```python
from build123d import *

# Parameters (mm, degrees)
F0_W     = 73.152
F0_H     = 76.2
F1_DEPTH = 22.352
F2_SIZE  = 25.4
F3_SIZE  = 6.35


with BuildPart() as f1:
    # F0 (on Right) → F1 (new body)
    with BuildSketch(Plane.YZ):
        with Locations((36.576, -38.1)):
            Rectangle(F0_W, F0_H)
    extrude(amount=F1_DEPTH)

    # F2
    f2_edges = [f1.edges().sort_by_distance(p)[0] for p in [
        (11.176, 0, -76.2),
        (11.176, 73.152, -76.2),
    ]]
    chamfer(f2_edges, length=F2_SIZE)

    # F3
    f3_edges = [f1.edges().sort_by_distance(p)[0] for p in [
        (0, 36.576, 0),
        (22.352, 36.576, 0),
    ]]
    chamfer(f3_edges, length=F3_SIZE)


solid = f1.part
```
Verification items for the finished model (mm, model axes). Round coordinates to 2 decimals unless told otherwise and drop trailing zeros. Order: outer loops, then holes, each group sorted by start corner. A loop starts at its lowest first (then second) coordinate and runs counter-clockwise, first axis right, second up. Notation, with made-up numbers: (8.25, -19.75) - (46.25, -19.75) arc R27 ccw to (46.25, 0.25) - close; hole circle Ø9 at (-13, 35). An arc over 180 degrees is marked (long way). Use CSV: the item, a comma, the result in double quotes.
(1) Mould release check, pull along Y, two halves, no side actions. Record for faces 1 (the face through (11.02, 60.63, -63.32)), 2 (the face through (11, 12.9, -63.7)), 3 (the face through (0, 36, -33)): released by +Y, released by -Y, zero draft, split by the parting line, or undercut.
Entries:
face 1,"released by +Y"
face 2,"released by -Y"
face 3,"zero draft"
(2) Section check B-B on x = 10. Record the boundary of the cut face in (y, z), and give its area (3 significant figures).
Entries:
outline,"(0, -50.8) - (25.4, -76.2) - (47.75, -76.2) - (73.15, -50.8) - (73.15, 0) - (0, 0) - close"
area,"4,930 mm^2"
(3) Section check D-D on z = -55. Record the boundary of the cut face in (x, y).
Entries:
outline,"(0, 4.2) - (22.35, 4.2) - (22.35, 68.95) - (0, 68.95) - close"
(4) Thickness scan on probe 1 along Z at (x, y) = (18.75, 32); probe 2 along Y at (x, z) = (18.5, -61); probe 3 along Z at (x, y) = (9.5, 66). Record the ranges inside material, lowest first. Write a range as from..to.
Entries:
probe 1,"-76.2..-2.75"
probe 2,"10.2..62.95"
probe 3,"-57.95..0"
(5) Section check A-A on y = 20.5. Record the boundary of the cut face in (x, z), and give its area (3 significant figures).
Entries:
outline,"(0, -71.3) - (22.35, -71.3) - (22.35, -6.35) - (16, 0) - (6.35, 0) - (0, -6.35) - close"
area,"1,550 mm^2"
(6) Gauge pin test, flat end, axial feed: pin 1 Ø1 at (x, z) = (7.5, -64) entering from +Y. Record the tip position at first contact, or that the pin passes through.
Entries:
pin 1,"y = 60.45"
(7) Section check C-C on z = -64. Record the boundary of the cut face in (x, y).
Entries:
outline,"(0, 13.2) - (22.35, 13.2) - (22.35, 59.95) - (0, 59.95) - close"
